Verification items for the finished model (mm, model axes). Give positions to 0.01 mm unless a question says otherwise; leave off trailing zeros. Loops run counter-clockwise (first coordinate to the right, second up) from the corner with the lowest first, then second, coordinate; pieces in that order, holes last. Notation, with made-up numbers: (-8.5, 41.25) - (32.5, 41.25) arc R30 ccw to (32.5, 71.25) - close; hole circle Ø2 at (-36, -9). An arc over 180 degrees is marked (long way). One line per question, with ' | ' between items. Start each with the question number.
1. Depth check by flat-ended pin: pin 1 Ø1.5 at (y, z) = (-33, 1.5) entering from +X; pin 2 Ø1.5 at (x, z) = (21.5, 2) entering from +Y; pin 3 Ø1.5 at (y, z) = (-32.5, 2) entering from -X. Enter the tip coordinate at first touch or a pass-through.
2. Section check D-D, the plane z = 2.3. State how many separate pieces and enclosed holes the cut face has, then the cut area to 3 significant figures.
3. Section check C-C, the plane x = 36.5. Enter the section's corners in (y, z), then the cut area to 3 significant figures.
4. Section check B-B, the plane y = 9. Enter the section's corners in (x, z), then the cut area to 3 significant figures.
5. Section check A-A, the plane x = 19. Enter the section's corners in (y, z).
6. Thickness scan on line 1 along Y through (x, z) = (-15, 1.1); line 2 along X through (y, z) = (0, 1.8); line 3 along X through (y, z) = (-6.5, 1.05). Record the ranges inside material, lowest first. Write a range as from..to.
from build123d import *

# Parameters (mm, degrees)
SKETCH1_W           = 85
SKETCH1_H           = 63
BOSS_EXTRUDE1_DEPTH = 3
SKETCH2_W           = 20
SKETCH2_H           = 3
CUT_EXTRUDE1_DEPTH  = 53.985847167
BOSS_EXTRUDE2_DEPTH = 3
SKETCH4_W           = 25
SKETCH4_H           = 3
BOSS_EXTRUDE3_DEPTH = 3


with BuildPart() as part:
    # Sketch1 → Boss-Extrude1 (new body)
    with BuildSketch(Plane.XY):
        Rectangle(SKETCH1_W, SKETCH1_H)
    extrude(amount=BOSS_EXTRUDE1_DEPTH)

    # Sketch2 → Cut-Extrude1 (cut, through all)
    with BuildSketch(Plane.XY.offset(3)):
        with Locations((-22.5, 0)):
            Rectangle(SKETCH2_W, SKETCH2_H)
        with Locations((22.5, 0)):
            Rectangle(SKETCH2_W, SKETCH2_H)
        with Locations((-22.5, -22)):
            Rectangle(SKETCH2_W, SKETCH2_H)
        with Locations((22.5, -22)):
            Rectangle(SKETCH2_W, SKETCH2_H)
    extrude(amount=-CUT_EXTRUDE1_DEPTH, mode=Mode.SUBTRACT)

    # Sketch3 → Boss-Extrude2 (add)
    with BuildSketch(Plane.XY.offset(3)):
        Polygon((-42.5, 31.5), (-48.5, 31.5), (-48.5, -31.5), (-42.5, -31.5), (-42.5, -10), (-45.5, -10), (-45.5, 10), (-42.5, 10), align=None)
        Polygon((42.5, 10), (42.5, 31.5), (48.5, 31.5), (48.5, -31.5), (42.5, -31.5), (42.5, -10), (45.5, -10), (45.5, 10), align=None)
    extrude(amount=-BOSS_EXTRUDE2_DEPTH)

    # Sketch4 → Boss-Extrude3 (add)
    with BuildSketch(Plane.XY.offset(3)):
        with Locations((0, 33)):
            Rectangle(SKETCH4_W, SKETCH4_H)
        with Locations((0, -33)):
            Rectangle(SKETCH4_W, SKETCH4_H)
    extrude(amount=-BOSS_EXTRUDE3_DEPTH)


solid = part.part
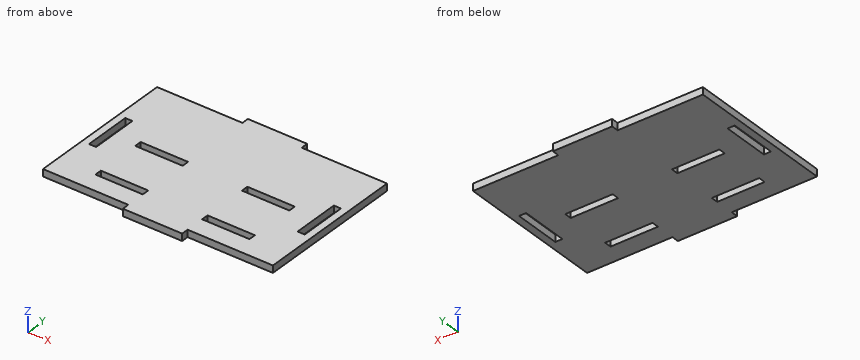
Results list:
1) pin 1: x = 12.5 | pin 2: y = 31.5 | pin 3: x = -12.5
2) separate pieces: 1 | enclosed holes: 6 | area: 5,900 mm²
3) outline: (-31.5, 0) - (31.5, 0) - (31.5, 3) - (-31.5, 3) - close | area: 189 mm²
4) outline: (-48.5, 0) - (-45.5, 0) - (-45.5, 3) - (-48.5, 3) - close; (-42.5, 0) - (42.5, 0) - (42.5, 3) - (-42.5, 3) - close; (45.5, 0) - (48.5, 0) - (48.5, 3) - (45.5, 3) - close | area: 273 mm²
5) outline: (-31.5, 0) - (-23.5, 0) - (-23.5, 3) - (-31.5, 3) - close; (-20.5, 0) - (-1.5, 0) - (-1.5, 3) - (-20.5, 3) - close; (1.5, 0) - (31.5, 0) - (31.5, 3) - (1.5, 3) - close
6) line 1: -31.5..-23.5, -20.5..-1.5, 1.5..31.5 | line 2: -48.5..-45.5, -42.5..-32.5, -12.5..12.5, 32.5..42.5, 45.5..48.5 | line 3: -48.5..-45.5, -42.5..42.5, 45.5..48.5
